```python
from build123d import *

# Parameters (mm, degrees)
F2_T     = -5.08
F3_R     = 3.81
F4_DEPTH = 304.8


# Not quite as in the source:
# - a feature names something its author has since deleted; it is built from what else it names


with BuildPart() as f1:
    # F0 (on Front) → F1 (revolve)
    with BuildSketch(Plane.XZ):
        Polygon((0, 0), (0, 63.5), (-38.1, 63.5), (-26.903236725, 0), align=None)
    revolve(axis=Axis((0, 0, 31.75), (0, 0, 1)))

    # F2
    f2_openings = [f1.faces().sort_by_distance(p)[0] for p in [
        (0, 0, 63.5),
    ]]
    offset(amount=F2_T, openings=f2_openings)

    # F3 (on Front) → F4 (cut)
    with BuildSketch(Plane.XZ):
        with Locations((0, 51.8186431976)):
            Circle(F3_R)
    extrude(amount=-F4_DEPTH, mode=Mode.SUBTRACT)


solid = f1.part
```
Model file for the job. Use its own axes, mm. A direction names the side the tool comes from. Give positions to 0.01 mm unless a question says otherwise; leave off trailing zeros. Loops run counter-clockwise (first coordinate to the right, second up) from the corner with the lowest first, then second, coordinate; pieces in that order, holes last. Notation, with made-up numbers: (31, -16.5) -> (46, -16.5) arc R10 ccw to (46, -1.5) -> close; hole circle Ø1 at (-22, 26). An arc over 180 degrees is marked (long way). Use CSV: the item, a comma, the result in double quotes. Start each with the question number.
1) Slice it at B-B on x = 0. Give the cut face in (y, z).
2) Mould opens along X. For faces 3 (the conical face through (6.759, 30.438, 24.25)), 4 (the flat face through (-17.1, -28.4, 63.5)), 5 (the cylindrical face through (2.05, 33.42, 55.03)) say: released by +X, released by -X, zero draft, split by the parting line, or undercut.
3) Tool access for faces 1 (the flat face through (0, 0, 0)), 2 (the flat face through (0, 0, 5.08)): list every direction of +Z, -Z, +X, -X, +Y, -Y with a clear straight run to the whole face (end or side of a thin tool).
4) Slice it at D-D on z = 38. Give the cut face in (x, y).
5) Wall check: line 1 (X direction, y = 7.5, z = 20.5); line 2 (Y direction, x = -22.5, z = 37); line 3 (Y direction, x = 16, z = 12). Give the ranges that are in metal, low to high.
6) Flat gauge pins, fed straight in: pin 1 Ø12 at (x, y) = (-4, -27) entering from -Z; pin 2 Ø6 at (x, y) = (-3, 10.5) entering from +Z; pin 3 Ø6 at (y, z) = (-18, 35.5) entering from +X; pin 4 Ø7 at (x, z) = (0, 51.82) entering from -Y. Where does each tip first touch, or does it go through?
7) Slice it at A-A on y = 0. Give the cut face in (x, z), plus the area to 3 significant figures.
8) Slice it at C-C on z = 58. Give the cut face in (x, y).
Computed values:
1,outline,"(-38.1, 63.5) -> (-26.9, 0) -> (26.9, 0) -> (35.37, 48.01) -> (30.21, 48.01) -> (22.64, 5.08) -> (-22.64, 5.08) -> (-32.94, 63.5) -> close; (31.55, 55.63) -> (36.71, 55.63) -> (38.1, 63.5) -> (32.94, 63.5) -> close"
2,face 3,"split by the parting line"
2,face 4,"zero draft"
2,face 5,"undercut"
3,face 1,"-Z, +X, -X, +Y, -Y"
3,face 2,"+Z"
4,outline,"circle Ø67.21 at (0, 0); hole circle Ø56.89 at (0, 0)"
5,line 1,"x = -29.58 to -24.23, 24.23 to 29.58"
5,line 2,"y = -24.72 to -17.11, 17.11 to 24.72"
5,line 3,"y = -24.21 to -17.7, 17.7 to 24.21"
6,pin 1,"stops at z = 0"
6,pin 2,"stops at z = 5.08"
6,pin 3,"stops at x = 29.69"
6,pin 4,"stops at y = -36.66"
7,outline,"(-38.1, 63.5) -> (-26.9, 0) -> (26.9, 0) -> (38.1, 63.5) -> (32.94, 63.5) -> (22.64, 5.08) -> (-22.64, 5.08) -> (-32.94, 63.5) -> close"
7,area,"881 mm^2"
8,outline,"circle Ø74.26 at (0, 0); hole circle Ø63.94 at (0, 0)"
